Could you check a few things on this model? Use its own coordinates, in mm. Coordinates: 2 decimals unless noted, no trailing zeros. Loops run counter-clockwise (first coordinate to the right, second up) from the corner with the lowest first, then second, coordinate; pieces in that order, holes last. Notation, with made-up numbers: M 17,81 L 36,81 A34 cw 36,115 Z; hole C 17,-17 d8. An arc over 180 degrees is marked long. Return JSON: item names as keys, results as strings. Group by question number.
from build123d import *

# Parameters (mm, degrees)
F0_R     = 1.75
F1_DEPTH = 0.75
F2_SIZE  = 0.2
F3_R     = 16
F4_DEPTH = 0.25


with BuildPart() as f1:
    # F0 (on Top) → F1 (new body, symmetric)
    with BuildSketch(Plane.XY):
        with BuildLine():
            ThreePointArc((-1.1283810214, 13.4527601729), (0.5269824002, 15.090801488), (2.0640494537, 13.3412780442))
            ThreePointArc((2.0640494537, 13.3412780442), (2.7028519806, 12.7159188095), (3.5407836432, 13.0273885024))
            ThreePointArc((3.5407836432, 13.0273885024), (5.6565595606, 14.000476204), (6.5025578694, 11.83075404))
            ThreePointArc((6.5025578694, 11.83075404), (6.888950435, 11.02462525), (7.7828775441, 11.0307215147))
            ThreePointArc((7.7828775441, 11.0307215147), (9.5873041905, 11.5334676573), (10.6323680347, 9.9789417592))
            Line((10.6323680347, 9.9789417592), (10.6003916286, 9.0234121058))
            ThreePointArc((10.6003916286, 9.0234121058), (11.2882923094, 8.300097914), (12, 9))
            Line((12, 9), (12, 15.8830052443))
            ThreePointArc((12, 15.8830052443), (-2.2823101594, 21.1363840676), (-14.5, 12.0638746292))
            Line((-14.5, 12.0638746292), (-14.5, 6.5256753509))
            ThreePointArc((-14.5, 6.5256753509), (-13.7743246491, 5.8), (-13.0486492981, 6.5256753509))
            Line((-13.0486492981, 6.5256753509), (-13.0486492981, 7.1539100671))
            ThreePointArc((-13.0486492981, 7.1539100671), (-12.082392441, 8.6230491446), (-10.3506872621, 8.3177310875))
            ThreePointArc((-10.3506872621, 8.3177310875), (-10.0687469644, 8.2680220118), (-9.9114299169, 8.5072137136))
            Line((-9.9114299169, 8.5072137136), (-9.9114299169, 10.6381451737))
            ThreePointArc((-9.9114299169, 10.6381451737), (-8.8408160288, 12.1480293893), (-7.0617419862, 11.6372848416))
            ThreePointArc((-7.0617419862, 11.6372848416), (-6.2563808661, 11.4060781626), (-5.7717294241, 12.0895809365))
            Line((-5.7717294241, 12.0895809365), (-5.7717294241, 12.83926297))
            ThreePointArc((-5.7717294241, 12.83926297), (-4.3750702496, 14.42628928), (-2.6234137882, 13.24264702))
            ThreePointArc((-2.6234137882, 13.24264702), (-1.8092503125, 12.8734848936), (-1.1283810214, 13.4527601729))
        make_face()
        with Locations((0, 19)):
            Circle(F0_R, mode=Mode.SUBTRACT)
    extrude(amount=F1_DEPTH, both=True)

    # F2
    f2_edges = [f1.edges().sort_by_distance(p)[0] for p in [
        (-1.75, 19, -0.75),
    ]]
    chamfer(f2_edges, length=F2_SIZE)

    # F3 (on Top) → F4 (cut, symmetric)
    with BuildSketch(Plane.XY):
        Circle(F3_R)
    extrude(amount=F4_DEPTH, both=True, mode=Mode.SUBTRACT)


solid = f1.part
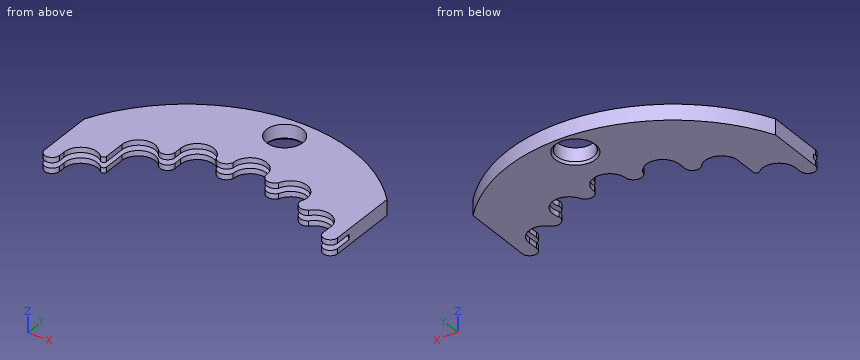
(1) Imagine slicing it at C-C, the plane y = 7.75. Write out the boundary of the cut face in (x, z), then the cut area to 3 significant figures.
(2) Imagine slicing it at D-D, the plane y = 16.5. Write out the boundary of the cut face in (x, z), then the cut area to 3 significant figures.
(3) Imagine slicing it at A-A, the plane x = 0. Write out the boundary of the cut face in (y, z).
(4) If I drill on L1, parallel to Y at x = 0, z = 0.2; L2, parallel to Z at x = -8, y = 13.25; L3, parallel to Y at x = 0, z = 0.3, over which ranges is the centre line in solid material (lowest first)? Write a range as [from, to].
(5) Imagine slicing it at B-B, the plane x = 11.3. Write out the boundary of the cut face in (y, z).
Checks:
{
 "1": {"outline": "M -14.5,-0.75 L -12.93,-0.75 L -12.93,-0.25 L -14,-0.25 L -14,0.25 L -12.93,0.25 L -12.93,0.75 L -14.5,0.75 Z", "area": "1.82 mm²"},
 "2": {"outline": "M -11.43,-0.75 L 11.43,-0.75 L 11.43,0.75 L -11.43,0.75 Z", "area": "34.3 mm²"},
 "3": {"outline": "M 15.02,-0.75 L 17.05,-0.75 L 17.25,-0.55 L 17.25,0.75 L 15.02,0.75 L 15.02,0.25 L 16,0.25 L 16,-0.25 L 15.02,-0.25 Z; M 20.75,-0.55 L 20.95,-0.75 L 21.3,-0.75 L 21.3,0.75 L 20.75,0.75 Z"},
 "4": {"L1": "[16, 17.25], [20.75, 21.3]", "L2": "[-0.75, -0.25], [0.25, 0.75]", "L3": "[15.02, 17.25], [20.75, 21.3]"},
 "5": {"outline": "M 8.3,-0.75 L 16.63,-0.75 L 16.63,0.75 L 8.3,0.75 L 8.3,0.25 L 11.33,0.25 L 11.33,-0.25 L 8.3,-0.25 Z"}
}
